Here's how the part is built. I have some questions about the finished solid (model axes, mm). Face numbers are marked on the shaded views. Coordinates: 2 decimals unless noted, no trailing zeros. Order: outer loops, then holes, each group sorted by start corner. A loop starts at its lowest first (then second) coordinate and runs counter-clockwise, first axis right, second up. Notation, with made-up numbers: (-3.5, -21) - (8.5, -21) arc R32 cw to (8.5, 5) - close; hole circle Ø4 at (51.5, -12). An arc over 180 degrees is marked (long way). Answer in a Markdown table with one row per item. Add a question column.
Item 1: Thinking about a two-plate mould opening in Y: for the marked faces 1, 2 and 3, which applies, +Y half, -Y half, draft (parallel to the pull), parting line (faces both ways), or undercut?
Item 2: I want a section at B-B (x = 273.25). Please give me the cut outline in (y, z), plus the area to 3 significant figures.
Item 3: I want a section at D-D (z = 2.25). Please give me the cut outline in (x, y).
Item 4: I want a section at A-A (z = 8.25). Please give me the cut outline in (x, y), plus the area to 3 significant figures.
Item 5: I want a section at C-C (y = 8.5). Please give me the cut outline in (x, z), plus the area to 3 significant figures.
Item 6: If I drill on line 1 along Z through (x, y) = (258.5, 6); line 2 along Y through (x, z) = (266.5, 10.75); line 3 along Y through (x, z) = (258.5, 3.5), over which ranges is the centre line in solid material (lowest first)? Write a range as from..to.
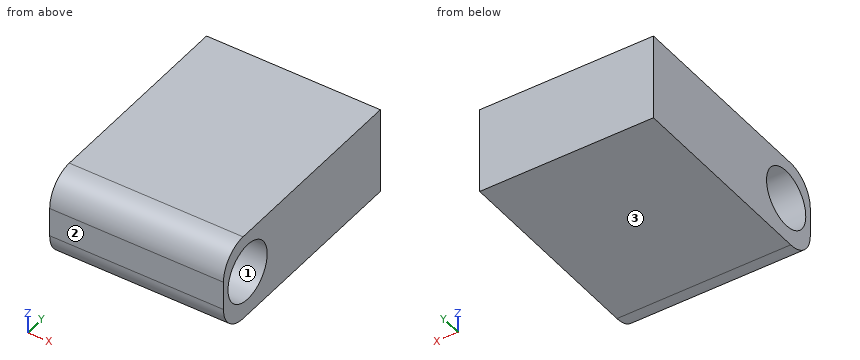
```python
from build123d import *

# Parameters (mm, degrees)
SKETCH1_W           = 30
SKETCH1_H           = 40
BOSS_EXTRUDE2_DEPTH = 15
FILLET4_R           = 5
FILLET5_R           = 5
SKETCH3_R           = 5
CUT_EXTRUDE2_DEPTH  = 53.201532545


with BuildPart() as part:
    # Sketch1 → Boss-Extrude2 (new body)
    with BuildSketch(Plane.XY):
        with Locations((271.793252061, 20)):
            Rectangle(SKETCH1_W, SKETCH1_H)
    extrude(amount=BOSS_EXTRUDE2_DEPTH)

    # Fillet4
    fillet4_edges = [part.edges().sort_by_distance(p)[0] for p in [
        (271.793252061, 0, 15),
    ]]
    fillet(fillet4_edges, radius=FILLET4_R)

    # Fillet5
    fillet5_edges = [part.edges().sort_by_distance(p)[0] for p in [
        (271.793252061, 0, 0),
    ]]
    fillet(fillet5_edges, radius=FILLET5_R)

    # Sketch3 → Cut-Extrude2 (cut, through all)
    with BuildSketch(Plane(origin=(286.793252061, 0, 0), x_dir=(0, 0, -1), z_dir=(1, 0, 0))):
        with Locations((-7.798550368, 6.154011522)):
            Circle(SKETCH3_R)
    extrude(amount=-CUT_EXTRUDE2_DEPTH, mode=Mode.SUBTRACT)


solid = part.part
```
Values follow:
| question | item | result |
|---|---|---|
| 1 | face 1 | undercut |
| 1 | face 2 | -Y half |
| 1 | face 3 | draft |
| 2 | outline | (0, 5) arc R5 ccw to (5, 0) - (40, 0) - (40, 15) - (5, 15) arc R5 ccw to (0, 10) - close; hole circle Ø10 at (6.15, 7.8) |
| 2 | area | 511 mm^2 |
| 3 | outline | (256.79, 0.82) - (286.79, 0.82) - (286.79, 40) - (256.79, 40) - close |
| 4 | outline | (256.79, 0) - (286.79, 0) - (286.79, 1.17) - (256.79, 1.17) - close; (256.79, 11.13) - (286.79, 11.13) - (286.79, 40) - (256.79, 40) - close |
| 4 | area | 901 mm^2 |
| 5 | outline | (256.79, 0) - (286.79, 0) - (286.79, 3.38) - (256.79, 3.38) - close; (256.79, 12.21) - (286.79, 12.21) - (286.79, 15) - (256.79, 15) - close |
| 5 | area | 185 mm^2 |
| 6 | line 1 | z = 0..2.8, 12.8..15 |
| 6 | line 2 | y = 0.06..2.12, 10.19..40 |
| 6 | line 3 | y = 0.23..3.6, 8.71..40 |
